Answer from the drawing. Dimensions are ordinates in mm from the lowest x, y and z of the part. A direction names the side the tool comes from. Give positions to 0.01 mm unless a question says otherwise; leave off trailing zeros. Loops run counter-clockwise (first coordinate to the right, second up) from the corner with the lowest first, then second, coordinate; pieces in that order, holes last. Notation, with made-up numbers: (55.5, -27) -> (85.5, -27) arc R32 cw to (85.5, 11) -> close; hole circle Ø10 at (-1.75, 33). An arc over 180 degrees is marked (long way). Write each question's results on one line, items separated by ' | '. Start each with the question number.
Item 1: Each of these flat-tipped pins is pushed along its axis until it touches: P1, Ø7, axis at x = 10.5, y = 26, coming from the +Z side; P2, Ø5, axis at y = 31.5, z = 12.5, coming from the -X side; P3, Ø5, axis at y = 8.5, z = 11, coming from the +X side. Where does it stop, or does it pass through?
Item 2: Section B-B on x = 7.5 is taken. Write down the section's boundary in (y, z).
Item 3: Find the intervals of material crossed by line 1 (X direction, y = 20.5, z = 9); line 2 (Z direction, x = 11, y = 16); line 3 (Z direction, x = 18.25, y = 22), in increasing order.
Item 4: Section A-A on y = 4 is taken. Write down the section's boundary in (x, z).
Item 5: Which of the six approach directions +Z, -Z, +X, -X, +Y, -Y give full straight-line access (tool end or side, diameter ignored) to the marked faces 1, 2 and 3?
Item 6: Section C-C on z = 8.25 is taken. Write down the section's boundary in (x, y).
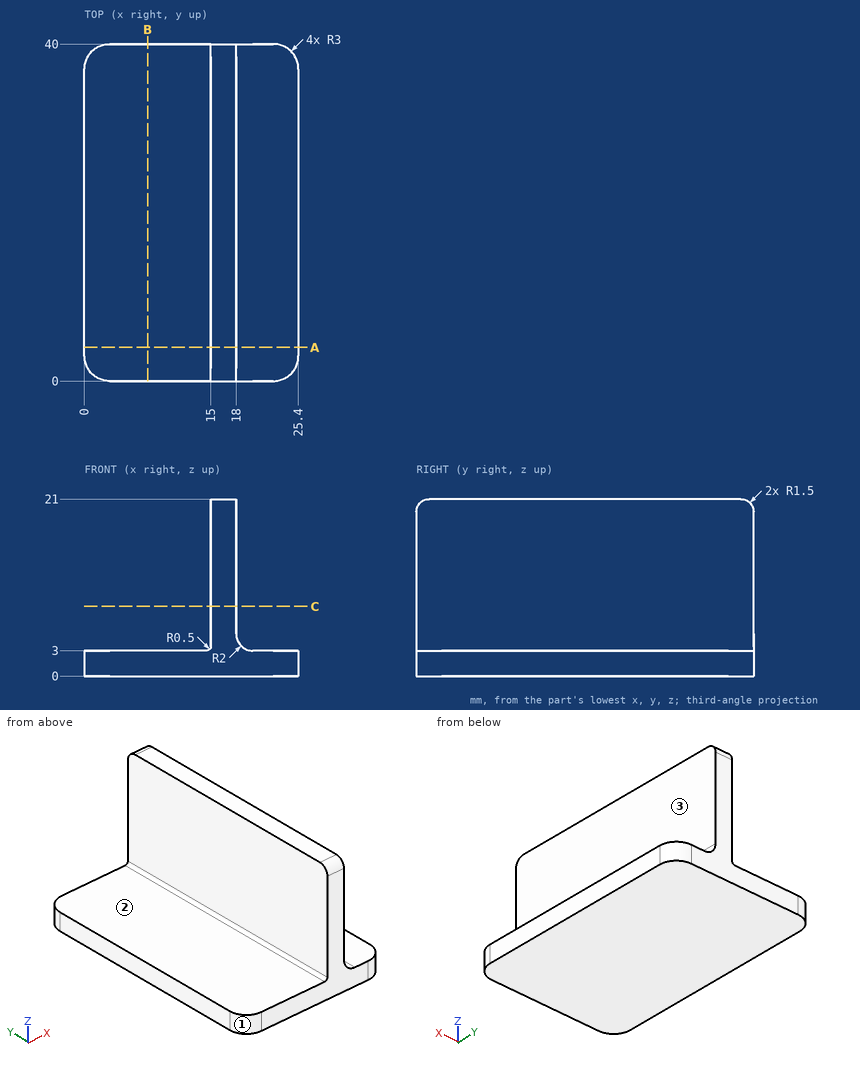
Findings:
1) P1: z = 3 | P2: x = 15 | P3: x = 18
2) outline: (0, 0) -> (40, 0) -> (40, 3) -> (0, 3) -> close
3) line 1: 15 to 18 | line 2: 0 to 3 | line 3: 0 to 4.03
4) outline: (0, 0) -> (25.4, 0) -> (25.4, 3) -> (20, 3) arc R2 cw to (18, 5) -> (18, 21) -> (15, 21) -> (15, 3.5) arc R0.5 cw to (14.5, 3) -> (0, 3) -> close
5) face 1: +Z, -Z, -X, -Y | face 2: +Z, -X, +Y, -Y | face 3: +Z, +X, +Y, -Y
6) outline: (15, 0) -> (18, 0) -> (18, 40) -> (15, 40) -> close
